Build history of the part. All positions in model axes, mm. Face numbers are marked on the shaded views. Round coordinates to 2 decimals unless told otherwise and drop trailing zeros. Write each loop counter-clockwise with the first axis right and the second up, starting at its lowest first coordinate (ties: lowest second). Pieces come first, ordered by that corner, then holes.
1) Pull direction Y, two halves, no side cores. Call the marked faces 1 and 2: +Y half, -Y half, draft (parallel to the pull), parting line (faces both ways), or undercut.
2) Flat gauge pin, fed straight in: pin 1 (8 mm diameter, centred on x = 42.5, z = 55, fed in from -Y). Where does the tip first touch, or does it go through?
3) Saw through at C-C (z = 145). Write the cut outline in (x, y).
4) Wall check: probe 1 along X at (y, z) = (-4.5, 190); probe 2 along Z at (x, y) = (125, -17.5); probe 3 along X at (y, z) = (-6, 145). Give the ranges that are in metal, low to high.
5) Saw through at B-B (x = 65). Write the cut outline in (y, z).
6) Saw through at A-A (z = 10). Write the cut outline in (x, y).
7) Saw through at D-D (y = -18). State how many separate pieces and enclosed holes the cut face has, plus the area to 3 significant figures.
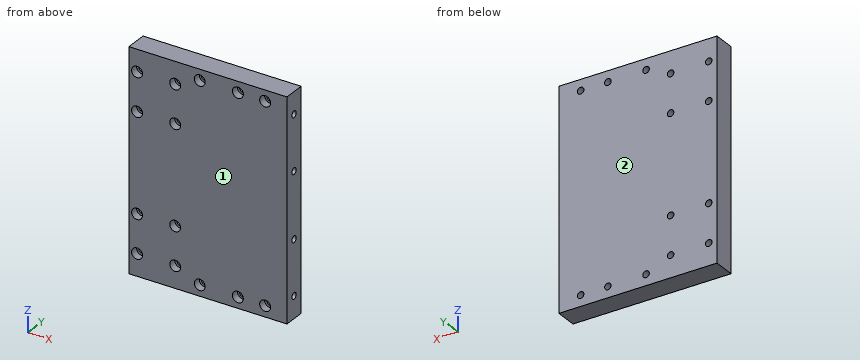
from build123d import *

# Parameters (mm, degrees)
F0_W     = 145
F0_H     = 200
F0_R     = 3
F1_DEPTH = 20
F2_R     = 5
F3_DEPTH = 7
F4_R     = 3
F5_DEPTH = 30
F6_R     = 3
F7_DEPTH = 20
F8_R     = 5
F9_DEPTH = 7


with BuildPart() as f1:
    # F0 (on Front) → F1 (new body)
    with BuildSketch(Plane.XZ):
        with Locations((72.5, 100)):
            Rectangle(F0_W, F0_H)
        with Locations((7.5, 20)):
            Circle(F0_R, mode=Mode.SUBTRACT)
        with Locations((42.5, 20)):
            Circle(F0_R, mode=Mode.SUBTRACT)
        with Locations((7.5, 55)):
            Circle(F0_R, mode=Mode.SUBTRACT)
        with Locations((42.5, 55)):
            Circle(F0_R, mode=Mode.SUBTRACT)
        with Locations((7.5, 145)):
            Circle(F0_R, mode=Mode.SUBTRACT)
        with Locations((42.5, 145)):
            Circle(F0_R, mode=Mode.SUBTRACT)
        with Locations((7.5, 180)):
            Circle(F0_R, mode=Mode.SUBTRACT)
        with Locations((42.5, 180)):
            Circle(F0_R, mode=Mode.SUBTRACT)
    extrude(amount=F1_DEPTH)

    # F2 (on face) → F3 (cut)
    with BuildSketch(Plane.XZ.offset(20)):
        with Locations((7.5, 180)):
            Circle(F2_R)
        with Locations((42.5, 180)):
            Circle(F2_R)
        with Locations((7.5, 145)):
            Circle(F2_R)
        with Locations((42.5, 145)):
            Circle(F2_R)
        with Locations((7.5, 55)):
            Circle(F2_R)
        with Locations((42.5, 55)):
            Circle(F2_R)
        with Locations((7.5, 20)):
            Circle(F2_R)
        with Locations((42.5, 20)):
            Circle(F2_R)
    extrude(amount=-F3_DEPTH, mode=Mode.SUBTRACT)

    # F4 (on face) → F5 (cut)
    with BuildSketch(Plane.YZ.offset(145)):
        with Locations((-10, 20)):
            Circle(F4_R)
        with Locations((-10, 70)):
            Circle(F4_R)
        with Locations((-10, 130)):
            Circle(F4_R)
        with Locations((-10, 180)):
            Circle(F4_R)
    extrude(amount=-F5_DEPTH, mode=Mode.SUBTRACT)

    # F6 (on face) → F7 (cut)
    with BuildSketch(Plane.XZ.offset(20)):
        with Locations((125, 190)):
            Circle(F6_R)
        with Locations((100, 190)):
            Circle(F6_R)
        with Locations((65, 190)):
            Circle(F6_R)
        with Locations((125, 10)):
            Circle(F6_R)
        with Locations((100, 10)):
            Circle(F6_R)
        with Locations((65, 10)):
            Circle(F6_R)
    extrude(amount=-F7_DEPTH, mode=Mode.SUBTRACT)

    # F8 (on face) → F9 (cut)
    with BuildSketch(Plane.XZ.offset(20)):
        with Locations((65, 190)):
            Circle(F8_R)
        with Locations((100, 190)):
            Circle(F8_R)
        with Locations((125, 190)):
            Circle(F8_R)
        with Locations((65, 10)):
            Circle(F8_R)
        with Locations((100, 10)):
            Circle(F8_R)
        with Locations((125, 10)):
            Circle(F8_R)
    extrude(amount=-F9_DEPTH, mode=Mode.SUBTRACT)


solid = f1.part
Evaluation:
1. face 1: -Y half
1. face 2: +Y half
2. pin 1: stops at y = -13
3. outline: (0, -20) - (2.5, -20) - (2.5, -13) - (4.5, -13) - (4.5, 0) - (0, 0) - close; (10.5, -13) - (12.5, -13) - (12.5, -20) - (37.5, -20) - (37.5, -13) - (39.5, -13) - (39.5, 0) - (10.5, 0) - close; (45.5, -13) - (47.5, -13) - (47.5, -20) - (145, -20) - (145, 0) - (45.5, 0) - close
4. probe 1: x = 0 to 62, 68 to 97, 103 to 122, 128 to 145
4. probe 2: z = 0 to 5, 15 to 185, 195 to 200
4. probe 3: x = 0 to 4.5, 10.5 to 39.5, 45.5 to 145
5. outline: (-20, 0) - (0, 0) - (0, 7) - (-13, 7) - (-13, 5) - (-20, 5) - close; (-20, 15) - (-13, 15) - (-13, 13) - (0, 13) - (0, 187) - (-13, 187) - (-13, 185) - (-20, 185) - close; (-20, 195) - (-13, 195) - (-13, 193) - (0, 193) - (0, 200) - (-20, 200) - close
6. outline: (0, -20) - (60, -20) - (60, -13) - (62, -13) - (62, 0) - (0, 0) - close; (68, -13) - (70, -13) - (70, -20) - (95, -20) - (95, -13) - (97, -13) - (97, 0) - (68, 0) - close; (103, -13) - (105, -13) - (105, -20) - (120, -20) - (120, -13) - (122, -13) - (122, 0) - (103, 0) - close; (128, -13) - (130, -13) - (130, -20) - (145, -20) - (145, 0) - (128, 0) - close
7. separate pieces: 1
7. enclosed holes: 14
7. area: 27,900 mm2
